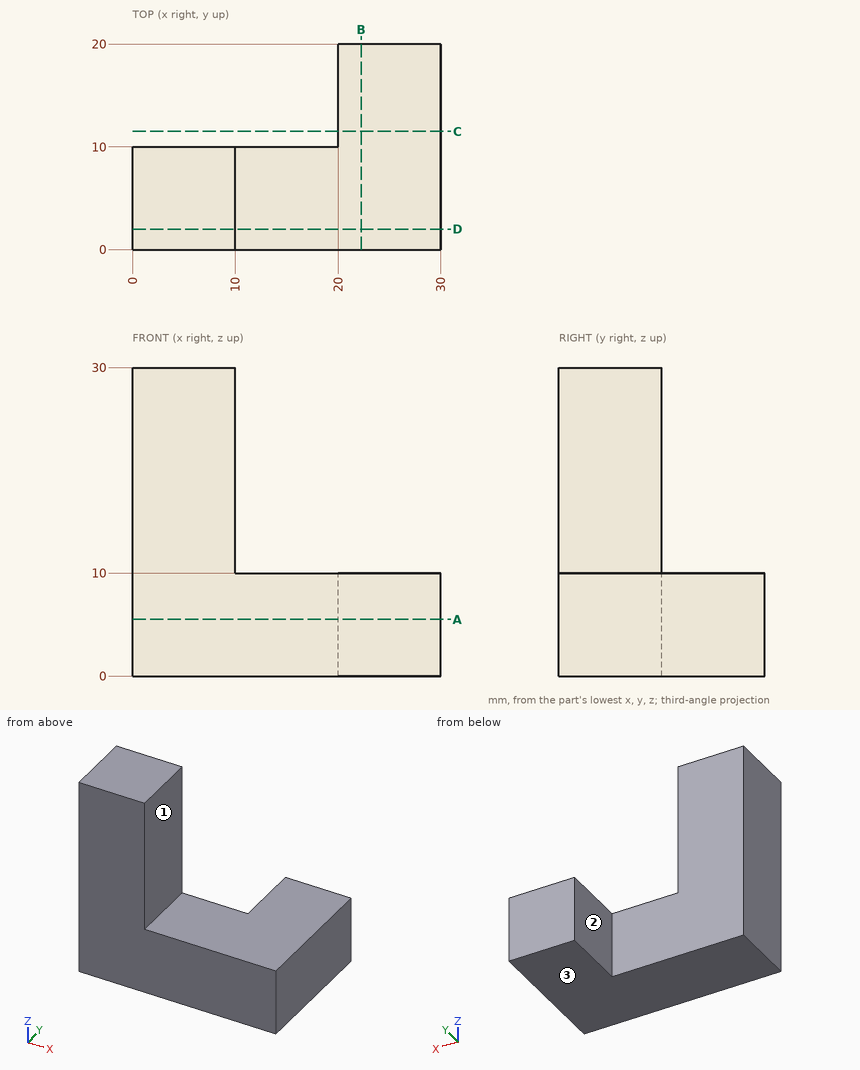
Print and shaded views of the part. All mm, measured from the part's lowest x, y and z. A direction names the side the tool comes from. Coordinates: 2 decimals unless noted, no trailing zeros. Loops run counter-clockwise (first coordinate to the right, second up) from the corner with the lowest first, then second, coordinate; pieces in that order, holes last. Notation, with made-up numbers: (58.5, 7) -> (80.5, 7) arc R22 ccw to (80.5, 24) -> close; hole circle Ø2 at (57.5, 61.25). An arc over 180 degrees is marked (long way). Use one line per item in the form item = value. Start each with the question number.
(1) Cut at C-C on y = 11.5. Give the cut face in (x, z).
(2) Cut at D-D on y = 2. Give the cut face in (x, z).
(3) Tool access for the marked faces 1, 2 and 3: list every direction of +Z, -Z, +X, -X, +Y, -Y with a clear straight run to the whole face (end or side of a thin tool).
(4) Flat gauge pins, fed straight in: pin 1 (8 mm diameter, centred on y = 15, z = 4.5, fed in from -X); pin 2 (6 mm diameter, centred on x = 7.5, z = 18, fed in from +Y); pin 3 (11 mm diameter, centred on y = 7.5, z = 24.5, fed in from +X). Where does each tip first touch, or does it go through?
(5) Cut at A-A on z = 5.5. Give the cut face in (x, y), and give its area (3 significant figures).
(6) Probe probe 1 along X at (y, z) = (1.25, 13.5); probe 2 along X at (y, z) = (13.75, 8). List the from-to ranges inside material, lowest first. Write a range as from..to.
(7) Cut at B-B on x = 22.25. Give the cut face in (y, z).
Values:
q1.outline = (20, 0) -> (30, 0) -> (30, 10) -> (20, 10) -> close
q2.outline = (0, 0) -> (30, 0) -> (30, 10) -> (10, 10) -> (10, 30) -> (0, 30) -> close
q3.face_1 = +Z, +X, +Y, -Y
q3.face_2 = +Z, -Z, -X, +Y
q3.face_3 = -Z, +X, -X, +Y, -Y
q4.pin_1 = 20
q4.pin_2 = 10
q4.pin_3 = 10
q5.outline = (0, 0) -> (30, 0) -> (30, 20) -> (20, 20) -> (20, 10) -> (0, 10) -> close
q5.area = 400 mm2
q6.probe_1 = 0..10
q6.probe_2 = 20..30
q7.outline = (0, 0) -> (20, 0) -> (20, 10) -> (0, 10) -> close
